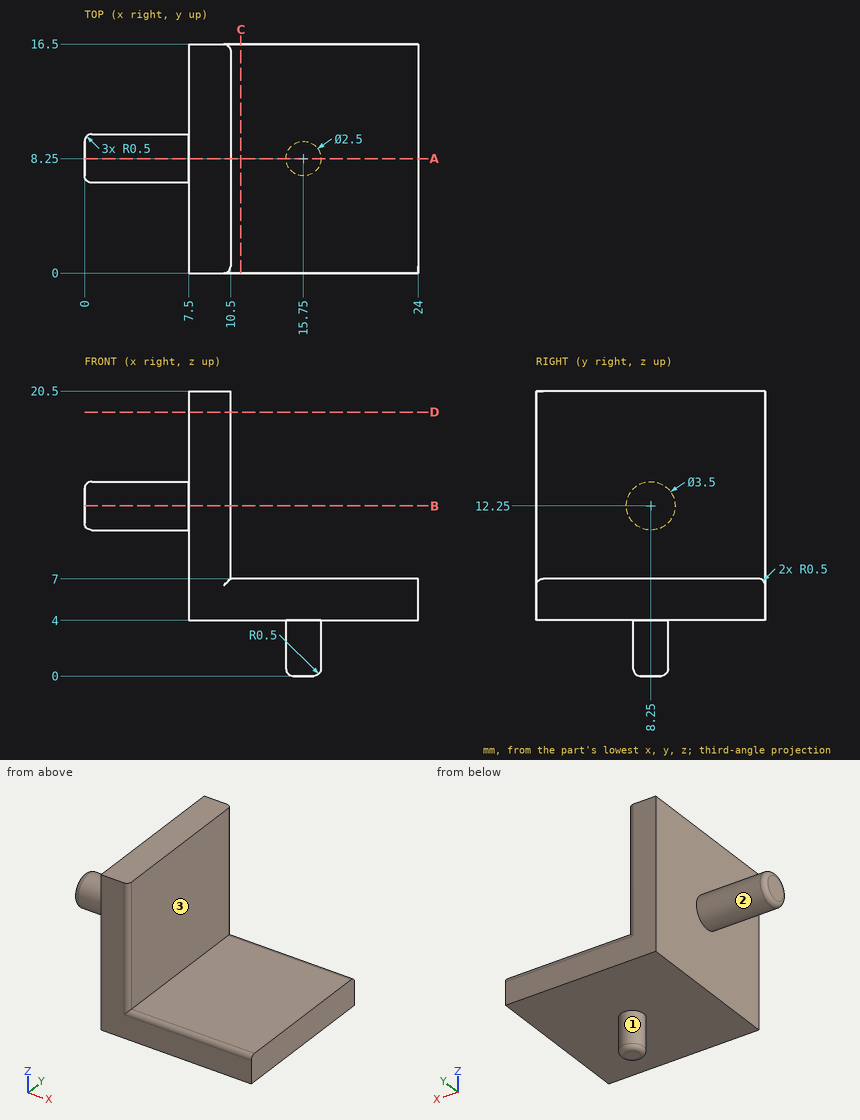
Study the drawing (mm; zero at the part's minimum x, y, z) and answer. A direction names the side the tool comes from. Coordinates: 2 decimals unless noted, no trailing zeros. Write each loop counter-clockwise with the first axis right and the second up, starting at its lowest first coordinate (ties: lowest second). Pieces come first, ordered by that corner, then holes. Notation, with made-up numbers: (88.5, 77) - (101.5, 77) arc R25 cw to (101.5, 92) - close; hole circle Ø11 at (20.5, -25). An arc over 180 degrees is marked (long way). Answer as a JSON object with one key per item and string values. Group by question number.
1. Which of the six approach directions +Z, -Z, +X, -X, +Y, -Y give full straight-line access (tool end or side, diameter ignored) to the marked faces 1, 2 and 3?
2. Consider L1, parallel to X at y = 2.5, z = 19; L2, parallel to Z at x = 8.25, y = 12; L3, parallel to Z at x = 13.5, y = 5.5. Determine where each line is inside the solid, lowest interval first. Write a range as [from, to].
3. A cutting plane is placed at C-C (x = 11.25). Determine the outline of the cut face in (y, z).
4. A cutting plane is placed at D-D (z = 19). Determine the outline of the cut face in (x, y).
5. A cutting plane is placed at A-A (y = 8.25). Determine the outline of the cut face in (x, z), plus the area to 3 significant figures.
6. Each of these flat-tipped pins is pushed along its axis until it touches: P1, Ø5, axis at y = 3, z = 8, coming from the -X side; P2, Ø4, axis at x = 16, y = 10.5, coming from the +Z side; P3, Ø5, axis at x = 11, y = 3.5, coming from the -Z side. Where does it stop, or does it pass through?
7. A cutting plane is placed at B-B (z = 12.25). Determine the outline of the cut face in (x, y).
Worked out:
{
 "1": {"face 1": "-Z", "face 2": "-X", "face 3": "+Z, +X, +Y, -Y"},
 "2": {"L1": "x = [7.5, 10.5]", "L2": "z = [4, 20.5]", "L3": "z = [4, 7]"},
 "3": {"outline": "(0, 4) - (16.5, 4) - (16.5, 6.5) arc R0.5 ccw to (16, 7) - (0.5, 7) arc R0.5 ccw to (0, 6.5) - close"},
 "4": {"outline": "(7.5, 0) - (10, 0) arc R0.5 ccw to (10.5, 0.5) - (10.5, 16) arc R0.5 ccw to (10, 16.5) - (7.5, 16.5) - close"},
 "5": {"outline": "(0, 11) arc R0.5 ccw to (0.5, 10.5) - (7.5, 10.5) - (7.5, 4) - (14.5, 4) - (14.5, 0.5) arc R0.5 ccw to (15, 0) - (16.5, 0) arc R0.5 ccw to (17, 0.5) - (17, 4) - (24, 4) - (24, 7) - (10.5, 7) - (10.5, 20.5) - (7.5, 20.5) - (7.5, 14) - (0.5, 14) arc R0.5 ccw to (0, 13.5) - close", "area": "126 mm²"},
 "6": {"P1": "stops at x = 7.5", "P2": "stops at z = 7", "P3": "stops at z = 4"},
 "7": {"outline": "(0, 7) arc R0.5 ccw to (0.5, 6.5) - (7.5, 6.5) - (7.5, 0) - (10, 0) arc R0.5 ccw to (10.5, 0.5) - (10.5, 16) arc R0.5 ccw to (10, 16.5) - (7.5, 16.5) - (7.5, 10) - (0.5, 10) arc R0.5 ccw to (0, 9.5) - close"}
}
